CAD build for the part. Positions are in the model's coordinates, mm. Coordinates: 2 decimals unless noted, no trailing zeros. Order: outer loops, then holes, each group sorted by start corner. A loop starts at its lowest first (then second) coordinate and runs counter-clockwise, first axis right, second up. Notation, with made-up numbers: (2, -30) - (15, -30) arc R13 ccw to (15, -5) - close; hole circle Ø1 at (-22.5, 24). An arc over 180 degrees is marked (long way). Write each question's results on one line, items separated by ' | '. Start each with the question number.
Q1. Wall check: probe 1 along X at (y, z) = (-0.25, 18.5); probe 2 along X at (y, z) = (-7.75, 23.25). Give the ranges that are in metal, low to high.
Q2. Band-saw the part on C-C, the plane z = 2. Write the cut outline in (x, y).
Q3. Band-saw the part on A-A, the plane x = 0. Write the cut outline in (y, z), then the cut area to 3 significant figures.
Q4. Pin check, flat tips, straight feed: P1, Ø1, axis at x = -1.5, z = 22, coming from the -Y side; P2, Ø2, axis at x = -2.5, z = 18, coming from the -Y side; P3, Ø6, axis at x = -5, z = 6, coming from the -Y side. Stop position of each tip, or through.
```python
from build123d import *

# Parameters (mm, degrees)
ESQUISSE1_R          = 12
ESQUISSE1_R_2        = 10
BASE_EXTRUSION_DEPTH = 30
CONG_1_R             = 0.5


with BuildPart() as part:
    # Esquisse1 → Base-Extrusion (new body)
    with BuildSketch(Plane.XY):
        Circle(ESQUISSE1_R)
        Circle(ESQUISSE1_R_2, mode=Mode.SUBTRACT)
    extrude(amount=BASE_EXTRUSION_DEPTH)

    # Congé1
    cong_1_edges = [part.edges().sort_by_distance(p)[0] for p in [
        (-12, 0, 0),
        (-12, 0, 30),
        (-10, 0, 0),
        (-10, 0, 30),
    ]]
    fillet(cong_1_edges, radius=CONG_1_R)


solid = part.part
```
Results below:
1) probe 1: x = -12 to -10, 10 to 12 | probe 2: x = -9.16 to -6.32, 6.32 to 9.16
2) outline: circle Ø24 at (0, 0); hole circle Ø20 at (0, 0)
3) outline: (-12, 0.5) arc R0.5 ccw to (-11.5, 0) - (-10.5, 0) arc R0.5 ccw to (-10, 0.5) - (-10, 29.5) arc R0.5 ccw to (-10.5, 30) - (-11.5, 30) arc R0.5 ccw to (-12, 29.5) - close; (10, 0.5) arc R0.5 ccw to (10.5, 0) - (11.5, 0) arc R0.5 ccw to (12, 0.5) - (12, 29.5) arc R0.5 ccw to (11.5, 30) - (10.5, 30) arc R0.5 ccw to (10, 29.5) - close | area: 120 mm²
4) P1: stops at y = -11.96 | P2: stops at y = -11.91 | P3: stops at y = -11.83
